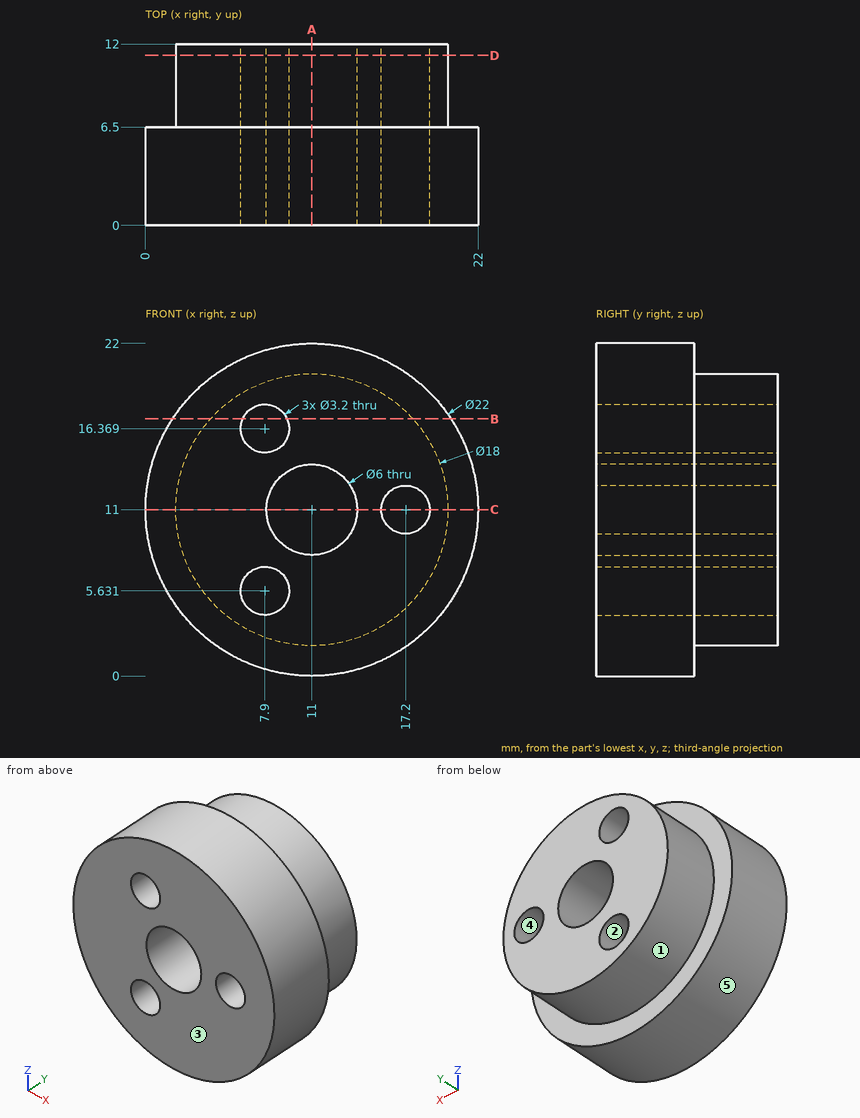
Source: three-view drawing plus pictorial views. Frame: mm from the lowest corner of the part. A direction names the side the tool comes from. Give positions to 0.01 mm unless a question says otherwise; leave off trailing zeros. Order: outer loops, then holes, each group sorted by start corner. A loop starts at its lowest first (then second) coordinate and runs counter-clockwise, first axis right, second up. Notation, with made-up numbers: M 26,8.5 L 74,8.5 A8 cw 74,16.5 Z; hole C 43.5,22.5 d8. An arc over 180 degrees is marked long. Return JSON: item names as keys, results as strings.
Item 1: First-contact query: P1, Ø1.5, axis at y = 3, z = 7.5, coming from the +X side; P2, Ø2, axis at y = 2, z = 19, coming from the -X side (1 decimal); P3, Ø4, axis at y = 10.5, z = 15.5, coming from the +X side. Flat tips, straight axial feed; report the tip coordinate or a pass-through.
Solutions:
{"P1": "x = 21.65", "P2": "x = 2.5", "P3": "x = 19.65"}
Item 2: Pull-direction query (Z, two-part tool) for the marked faces 3, 4 and 5; classes: +Z half, -Z half, draft (parallel to the pull), parting line (faces both ways), or undercut.
Solutions:
{"face 3": "draft", "face 4": "undercut", "face 5": "parting line"}
Item 3: Cut plane D-D (y = 11.25). Return loops of the section in (x, z) (1 decimal).
Solutions:
{"outline": "C 11,11 d18; hole C 7.9,5.6 d3.2; hole C 7.9,16.4 d3.2; hole C 11,11 d6; hole C 17.2,11 d3.2"}
Item 4: Cut plane A-A (x = 11). Return loops of the section in (y, z), then the cut area to 3 significant figures.
Solutions:
{"outline": "M 0,0 L 6.5,0 L 6.5,2 L 12,2 L 12,8 L 0,8 Z; M 0,14 L 12,14 L 12,20 L 6.5,20 L 6.5,22 L 0,22 Z", "area": "170 mm^2"}
Item 5: Cut plane C-C (z = 11). Return loops of the section in (x, y), then the cut area to 3 significant figures.
Solutions:
{"outline": "M 0,0 L 8,0 L 8,12 L 2,12 L 2,6.5 L 0,6.5 Z; M 14,0 L 15.6,0 L 15.6,12 L 14,12 Z; M 18.8,0 L 22,0 L 22,6.5 L 20,6.5 L 20,12 L 18.8,12 Z", "area": "132 mm^2"}
Item 6: Ray query, probe 1 along X at (y, z) = (4, 11); probe 2 along X at (y, z) = (7, 11); probe 3 along Z at (x, y) = (7.5, 9.5). Return the intervals inside material, ascending.
Solutions:
{"probe 1": "0 to 8, 14 to 15.6, 18.8 to 22", "probe 2": "2 to 8, 14 to 15.6, 18.8 to 20", "probe 3": "2.71 to 4.08, 7.18 to 14.82, 17.92 to 19.29"}
Item 7: Cut plane B-B (z = 17). Return loops of the section in (x, y).
Solutions:
{"outline": "M 1.78,0 L 6.43,0 L 6.43,12 L 4.29,12 L 4.29,6.5 L 1.78,6.5 Z; M 9.37,0 L 20.22,0 L 20.22,6.5 L 17.71,6.5 L 17.71,12 L 9.37,12 Z"}
Item 8: Access query for the marked faces 1 and 2. Directions: +Z, -Z, +X, -X, +Y, -Y. A direction counts if a zero-diameter tool reaches every point of the face in a straight line with its end or side. Return the directions, or none.
Solutions:
{"face 1": "+Y", "face 2": "+Y, -Y"}
